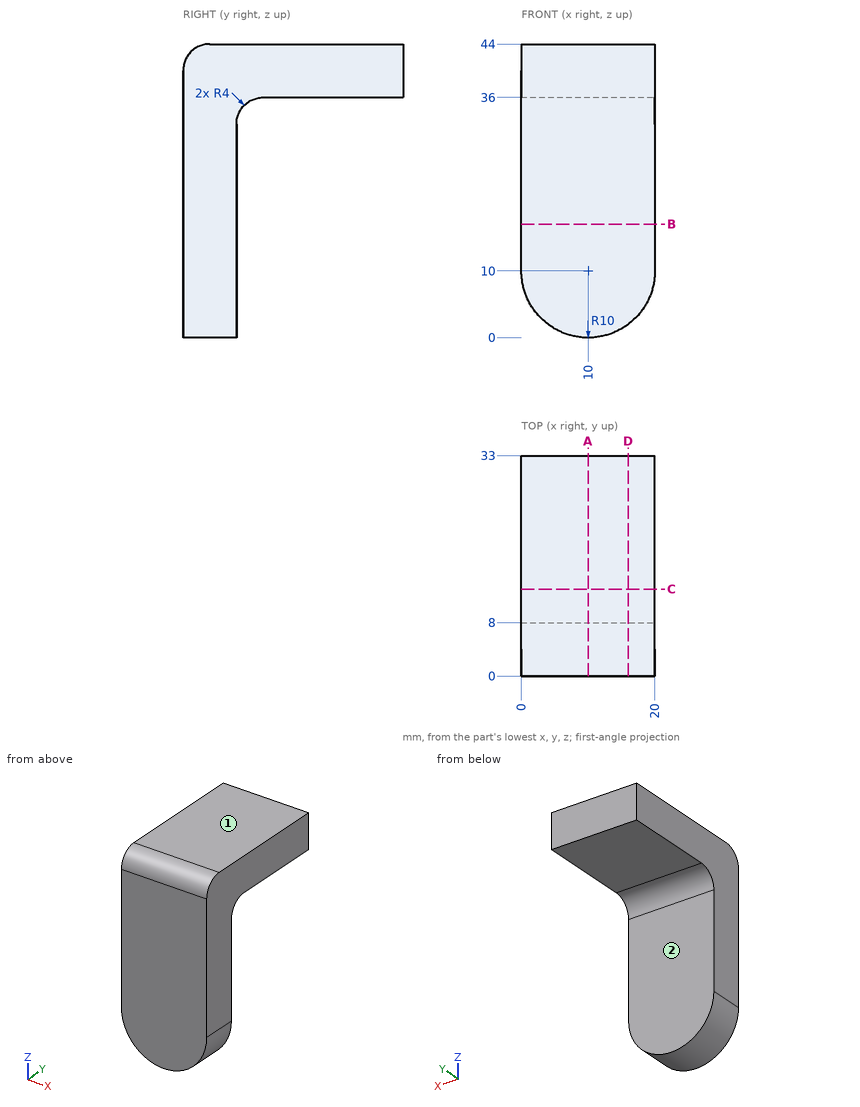
Part print with two shaded views. Sizes in mm from the minimum x, y, z corner. A direction names the side the tool comes from. Coordinates: 2 decimals unless noted, no trailing zeros. Loops run counter-clockwise (first coordinate to the right, second up) from the corner with the lowest first, then second, coordinate; pieces in that order, holes last. Notation, with made-up numbers: (39, 66) - (43, 66) arc R12 ccw to (43, 77) - close; hole circle Ø11 at (47, -31). An arc over 180 degrees is marked (long way). Write each question's results on one line, items separated by ' | '. Start each with the question number.
Q1. Slice it at C-C on y = 13. Give the cut face in (x, z).
Q2. Slice it at B-B on z = 17. Give the cut face in (x, y).
Q3. Which spindle directions (+Z, -Z, +X, -X, +Y, -Y) get a long thin tool onto all of the face, cutting with end or side? Do the marked faces 1 and 2. Say none if no direction does.
Q4. Probe line 1 along Z through (x, y) = (6.5, 21.5); line 2 along Y through (x, z) = (17, 20); line 3 along Z through (x, y) = (17.75, 2). List the from-to ranges inside material, lowest first.
Q5. Drop flat-ended pins along their axis: pin 1 Ø6 at (x, y) = (8.5, 25.5) entering from -Z; pin 2 Ø5 at (x, y) = (8.5, 6.5) entering from -Z; pin 3 Ø10 at (x, y) = (18, 5) entering from -Z. Give the stop position or say it passes through.
Q6. Slice it at A-A on x = 10. Give the cut face in (y, z), and give its area (3 significant figures).
Q7. Slice it at D-D on x = 16. Give the cut face in (y, z).
Answer:
1) outline: (0, 36) - (20, 36) - (20, 44) - (0, 44) - close
2) outline: (0, 0) - (20, 0) - (20, 8) - (0, 8) - close
3) face 1: +Z, +X, -X, +Y, -Y | face 2: -Z, +X, -X, +Y
4) line 1: z = 36 to 44 | line 2: y = 0 to 8 | line 3: z = 3.68 to 43.46
5) pin 1: stops at z = 36 | pin 2: stops at z = 0 | pin 3: stops at z = 0.46
6) outline: (0, 0) - (8, 0) - (8, 32) arc R4 cw to (12, 36) - (33, 36) - (33, 44) - (4, 44) arc R4 ccw to (0, 40) - close | area: 552 mm2
7) outline: (0, 2) - (8, 2) - (8, 32) arc R4 cw to (12, 36) - (33, 36) - (33, 44) - (4, 44) arc R4 ccw to (0, 40) - close
